from build123d import *

# Parameters (mm, degrees)
F3_DEPTH = 45.72
F4_COUNT = 12


with BuildPart() as f1:
    # F0 (on Front) → F1 (revolve)
    with BuildSketch(Plane.XZ):
        Polygon((44.45, 17.0215574244), (44.45, 42.4215574244), (-44.45, 42.4215574244), (-44.45, 17.0215574244), (-10.4945171624, 17.0215574244), (-10.4945171624, -13.4584425756), (-39.6297698409, -13.4584425756), (-39.6297698409, -38.8584425756), (-22.9390684722, -38.8584425756), (-22.9390684722, -42.6684425756), (-15.3190684722, -42.6684425756), (-15.3190684722, -38.8584425756), (-4.2934667461, -38.8584425756), (-4.2934667461, -55.5271957506), (4.2934667461, -55.5271957506), (4.2934667461, -38.8584425756), (19.6994334923, -38.8584425756), (19.6994334923, -42.6684425756), (27.3194334923, -42.6684425756), (27.3194334923, -38.8584425756), (39.6297698409, -38.8584425756), (39.6297698409, -13.4584425756), (12.710894458, -13.4584425756), (12.710894458, 17.0215574244), align=None)
    revolve(axis=Axis((2.7257320471, 0, -67.4719884992), (1, 0, 0)))

    # F2 (on Right) → F3 (cut, symmetric)
    with BuildSketch(Plane.YZ):
        Polygon((-13.5587146506, 23.0656899512), (13.5587146506, 23.0656899512), (24.6522054076, 48.3342073858), (-24.6522054076, 48.3342073858), align=None)
    f3 = extrude(amount=F3_DEPTH, both=True, mode=Mode.SUBTRACT)

    # F4: F3 ×12 about axis
    f4_axis = Axis((44.45, 0, -67.4719884992), (1, 0, 0))
    for i in range(1, F4_COUNT):
        add(f3.rotate(f4_axis, i * 360 / F4_COUNT), mode=Mode.SUBTRACT)


solid = f1.part
Part model, mm, in its own coordinate system. A direction names the side the tool comes from. Give positions to 0.01 mm unless a question says otherwise; leave off trailing zeros. Write each loop counter-clockwise with the first axis right and the second up, starting at its lowest first coordinate (ties: lowest second). Pieces come first, ordered by that corner, then holes.
1) Cut at A-A on z = -162. Write the cut outline in (x, y), then the cut area to 3 significant figures.
Resolved:
outline: (-44.45, -34.56) - (44.45, -34.56) - (44.45, -15.31) - (-44.45, -15.31) - close; (-44.45, 15.31) - (44.45, 15.31) - (44.45, 34.56) - (-44.45, 34.56) - close
area: 3,420 mm2
2) Cut at B-B on x = 17. State how many separate pieces and enclosed holes the cut face has, then the cut area to 3 significant figures.
Resolved:
separate pieces: 2
enclosed holes: 2
area: 14,200 mm2
3) Which spindle directions (+Z, -Z, +X, -X, +Y, -Y) get a long thin tool onto all of the face, cutting with end or side? Do faces 5 (the face through (-25.27, -16.22, -15.95)), 6 (the face through (39.63, 23, -91)), 7 (the face through (0.62, 99.31, -50.06)), 8 (the face through (0.62, -17.41, 31.84)). Say none if no direction does.
Resolved:
face 5: -X
face 6: +X
face 7: +X, -X, +Y
face 8: +Z, +X, -X
4) Pin check, flat tips, straight feed: pin 1 (1.5 mm diameter, centred on x = 19.5, y = 52, fed in from -Z); pin 2 (1.5 mm diameter, centred on x = -3.5, y = 49.5, fed in from +Z); pin 3 (17 mm diameter, centred on y = -0.5, z = -78.5, fed in from +X); pin 4 (10 mm diameter, centred on x = -4, z = -93.5, fed in from -Y). Stop position of each tip, or through.
Resolved:
pin 1: stops at z = -142.43
pin 2: stops at z = 8.93
pin 3: stops at x = 4.29
pin 4: stops at y = -107.84
5) Probe L1, parallel to Z at x = -11.25, y = 0; L2, parallel to Z at x = -21, y = 0; L3, parallel to Z at x = 2.25, y = 0. List the from-to ranges inside material, lowest first.
Resolved:
L1: z = -158.01 to -151.97, -121.49 to -96.09, -38.86 to -13.46, 17.02 to 23.07
L2: z = -158.01 to -151.97, -121.49 to -92.28, -42.67 to -13.46, 17.02 to 23.07
L3: z = -158.01 to -79.42, -55.53 to 23.07
6) Two-plate mould, pull along Z, no slides. Class faces 1 (the face through (0.62, -94.45, -102.02)), 2 (the face through (0.62, 17.3, 31.59)), 3 (the face through (0.62, 34.55, -161.92)), 4 (the face through (44.45, 55, -3)): released by +Z, released by -Z, zero draft, split by the parting line, or undercut.
Resolved:
face 1: released by -Z
face 2: released by +Z
face 3: undercut
face 4: zero draft
7) Cut at C-C on z = -128.5. Write the cut outline in (x, y).
Resolved:
outline: (-44.45, -74.58) - (44.45, -74.58) - (44.45, -58.44) - (12.71, -58.44) - (12.71, 58.44) - (44.45, 58.44) - (44.45, 74.58) - (-44.45, 74.58) - (-44.45, 58.44) - (-10.49, 58.44) - (-10.49, -58.44) - (-44.45, -58.44) - close
